Autodesk Inventor part; units mm, degrees
ref_plane "YZ Plane" through (0, 0, 0) normal (1, 0, 0) x (0, 1, 0)
ref_plane "XZ Plane" through (0, 0, 0) normal (0, 1, 0) x (-1, 0, 0)
ref_plane "XY Plane" through (0, 0, 0) normal (0, 0, 1) x (1, 0, 0)
sketch "Sketch1" plane through (0, 0, 0) normal (1, 0, 0) x (0, 1, 0)
  line L0 (0, 0) -> (-50.8, 0)
  line L1 (-50.8, 0) -> (-50.8, 3.175)
  line L2 (-50.8, 3.175) -> (0, 3.175)
  line L3 (0, 3.175) -> (0, 0)
  line L4 (0, 0) -> (25.4, 0)
  line L5 (25.4, 0) -> (25.4, 3.175)
  line L6 (25.4, 3.175) -> (0, 3.175)
  line L7 (0, 3.175) -> (0, 0)
  line L8 (0, 0) -> (25.4, 0) construction
  dimension "d0" = 50.8
  dimension "d1" = 3.175
  dimension "d2" = 25.4
  dimension "d3" = 0
  dimension "d4" = 3.175
extrude "Extrusion1" add sketch "Sketch1" along normal blind 76.2
sketch "Sketch2" plane through (76.2, 25.4, 0) normal (0, 0, -1) x (-1, 0, 0)
  line L0 (76.2, 0) -> (0, 0)
  line L1 (76.2, -76.2) -> (76.2, 0)
  line L2 (0, -76.2) -> (0, 0)
  line L3 (76.2, -76.2) -> (0, -76.2)
  point P0 (12.7, -12.7)
  point P1 (63.5, -12.7)
hole "Hole1" at (63.5, 12.7, 0) at (12.7, 12.7, 0) direction (0, 0, 1) diameter 6.35 end through all
sketch "Sketch3" plane through (0, -50.8, 0) normal (0, 0, -1) x (-1, 0, 0)
  line L0 (0, 0) -> (0, 76.2)
  line L1 (-76.2, 0) -> (-76.2, 76.2)
  line L2 (0, 0) -> (-76.2, 0)
  line L3 (0, 76.2) -> (-76.2, 76.2)
  point P0 (0, 50.8)
  point P1 (-38.1, 6.35)
  dimension "d18" = 6.35
  dimension "d19" = 38.1
hole "Hole2" at (38.1, -44.45, 0) direction (0, 0, 1) diameter 3.9688 end through all
properties part number "camera mount" material "Aluminum 6061"
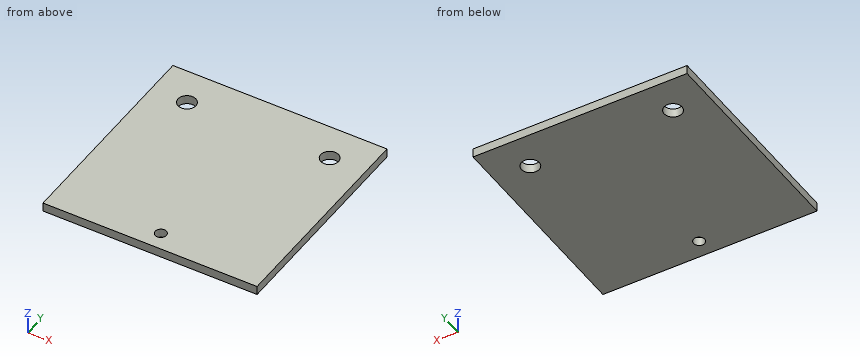
The listing builds one solid part. Answer for the finished solid, in the listing's coordinates (mm). Round coordinates to 2 decimals unless told otherwise and drop trailing zeros. Write each loop counter-clockwise with the first axis right and the second up, starting at its lowest first coordinate (ties: lowest second). Pieces come first, ordered by that corner, then holes. Notation, with made-up numbers: (16, 0.5) -> (49, 0.5) arc R4 ccw to (49, 6.5) -> close; hole circle Ø4 at (53.25, -7.75). An arc over 180 degrees is marked (long way). Use CSV: the item, a comma, the result in double quotes. Start each with the question number.
(1) Section A-A on y = -44.45 is taken. Give the vertices of the cut face in (x, z) (3 decimals), then the cut area to 3 significant figures.
(2) Section B-B on x = 38.1 is taken. Give the vertices of the cut face in (y, z) (3 decimals).
(3) Section C-C on y = 12.7 is taken. Give the vertices of the cut face in (x, z) (3 decimals).
(4) Consider L1, parallel to X at y = 12.7, z = 2.45 (3 decimals); L2, parallel to Y at x = 12.7, z = 2 (3 decimals); L3, parallel to X at y = 12, z = 0.35. Determine where each line is inside the solid, lowest interval first. Write a range as from..to.
A:
1,outline,"(0, 0) -> (36.116, 0) -> (36.116, 3.175) -> (0, 3.175) -> close; (40.084, 0) -> (76.2, 0) -> (76.2, 3.175) -> (40.084, 3.175) -> close"
1,area,"229 mm²"
2,outline,"(-50.8, 0) -> (-46.434, 0) -> (-46.434, 3.175) -> (-50.8, 3.175) -> close; (-42.466, 0) -> (25.4, 0) -> (25.4, 3.175) -> (-42.466, 3.175) -> close"
3,outline,"(0, 0) -> (9.525, 0) -> (9.525, 3.175) -> (0, 3.175) -> close; (15.875, 0) -> (60.325, 0) -> (60.325, 3.175) -> (15.875, 3.175) -> close; (66.675, 0) -> (76.2, 0) -> (76.2, 3.175) -> (66.675, 3.175) -> close"
4,L1,"x = 0..9.525, 15.875..60.325, 66.675..76.2"
4,L2,"y = -50.8..9.525, 15.875..25.4"
4,L3,"x = 0..9.6, 15.8..60.4, 66.6..76.2"
